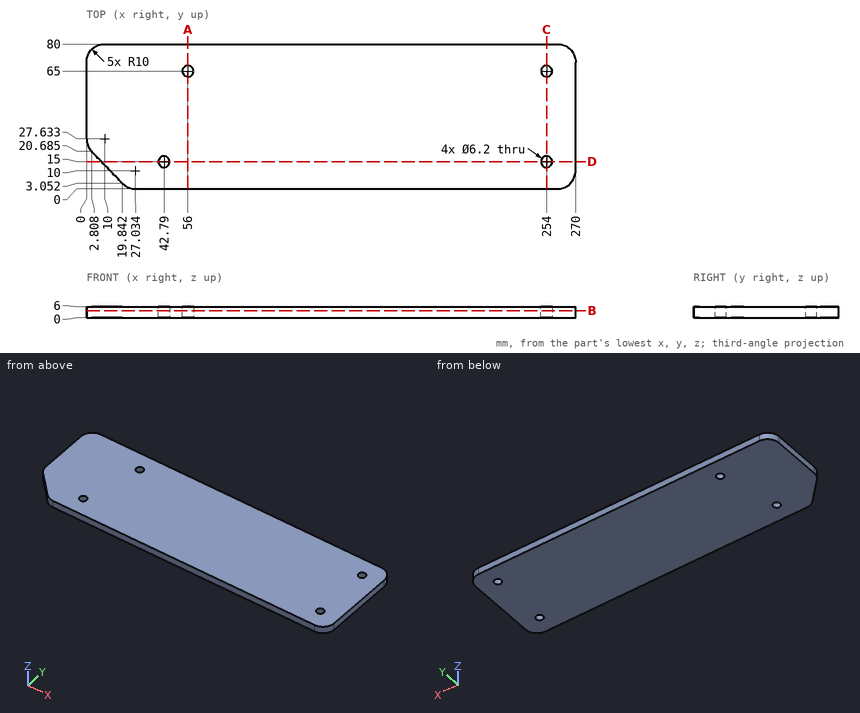
Could you check a few things on this drawing? It's one solid part, dimensions in mm from its lowest x, y, z. Give positions to 0.01 mm unless a question says otherwise; leave off trailing zeros. Order: outer loops, then holes, each group sorted by start corner. A loop starts at its lowest first (then second) coordinate and runs counter-clockwise, first axis right, second up. Notation, with made-up numbers: (30.5, 46.5) - (77.5, 46.5) arc R3 ccw to (77.5, 50.5) - close; hole circle Ø1 at (-1, -9.5). An arc over 180 degrees is marked (long way). Answer as a JSON object with one key per item and string values. Group by question number.
Item 1: If we section it at B-B on z = 3.95: Please give me the cut outline in (x, y) (1 decimal).
Item 2: If we section it at C-C on x = 254: Please give me the cut outline in (y, z).
Item 3: Please list where these lines run through material, in increasing order: probe 1 along X at (y, z) = (65.5, 4.15); probe 2 along Y at (x, z) = (254, 2.75); probe 3 along Y at (x, z) = (56, 4.7).
Item 4: For P1, Ø5.5, axis at x = 254, y = 15, coming from the +Z side, with a flat end and sliding along its axis, tell me the tip position at first contact or that it passes through.
Item 5: If we section it at D-D on y = 15: Please give me the cut outline in (x, z), and give its area (3 significant figures).
Item 6: If we section it at A-A on x = 56: Please give me the cut outline in (y, z), and give its area (3 significant figures).
Result set:
{
 "1": {"outline": "(0, 27.6) arc R10 ccw to (2.8, 20.7) - (19.8, 3.1) arc R10 ccw to (27, 0) - (260, 0) arc R10 ccw to (270, 10) - (270, 70) arc R10 ccw to (260, 80) - (10, 80) arc R10 ccw to (0, 70) - close; hole circle Ø6.2 at (42.8, 15); hole circle Ø6.2 at (56, 65); hole circle Ø6.2 at (254, 15); hole circle Ø6.2 at (254, 65)"},
 "2": {"outline": "(0, 0) - (11.9, 0) - (11.9, 6) - (0, 6) - close; (18.1, 0) - (61.9, 0) - (61.9, 6) - (18.1, 6) - close; (68.1, 0) - (80, 0) - (80, 6) - (68.1, 6) - close"},
 "3": {"probe 1": "0 to 52.94, 59.06 to 250.94, 257.06 to 270", "probe 2": "0 to 11.9, 18.1 to 61.9, 68.1 to 80", "probe 3": "0 to 61.9, 68.1 to 80"},
 "4": {"P1": "through"},
 "5": {"outline": "(8.3, 0) - (39.69, 0) - (39.69, 6) - (8.3, 6) - close; (45.89, 0) - (250.9, 0) - (250.9, 6) - (45.89, 6) - close; (257.1, 0) - (270, 0) - (270, 6) - (257.1, 6) - close", "area": "1,500 mm²"},
 "6": {"outline": "(0, 0) - (61.9, 0) - (61.9, 6) - (0, 6) - close; (68.1, 0) - (80, 0) - (80, 6) - (68.1, 6) - close", "area": "443 mm²"}
}
